from build123d import *

# Parameters (mm, degrees)
F1_DEPTH = 127
F2_R     = 33.02
F3_DEPTH = 121.92
F2_R_2   = 35.052
F4_DEPTH = 25.4
F5_R     = 2.54
F6_W     = 76.2
F6_H     = 2.54
F7_DEPTH = 5.08
F8_W     = 76.2
F8_H     = 2.54
F9_DEPTH = 5.08


with BuildPart() as f1:
    # F0 (on Top) → F1 (new body)
    with BuildSketch(Plane.XY):
        with BuildLine():
            Line((38.1, -33.553976), (18.048288, -33.553976))
            ThreePointArc((18.048288, -33.553976), (0, 38.1), (-18.048288, -33.553976))
            Line((-18.048288, -33.553976), (-38.1, -33.553976))
            Line((-38.1, -33.553976), (-38.1, -38.1))
            Line((-38.1, -38.1), (38.1, -38.1))
            Line((38.1, -38.1), (38.1, -33.553976))
        make_face()
    extrude(amount=F1_DEPTH)

    # F2 (on face) → F3 (cut)
    with BuildSketch(Plane.XY.offset(127)):
        Circle(F2_R)
    extrude(amount=-F3_DEPTH, mode=Mode.SUBTRACT)

    # F2 (on face) → F4 (join)
    with BuildSketch(Plane.XY.offset(127)):
        Circle(F2_R_2)
        Circle(F2_R, mode=Mode.SUBTRACT)
    extrude(amount=F4_DEPTH)

    # F5
    f5_edges = [f1.edges().sort_by_distance(p)[0] for p in [
        (18.048288, -33.553976, 63.5),
        (-18.048288, -33.553976, 63.5),
    ]]
    fillet(f5_edges, radius=F5_R)

    # F6 (on face) → F7 (join)
    with BuildSketch(Plane.XZ.offset(38.1)):
        with Locations((0, 1.27)):
            Rectangle(F6_W, F6_H)
    extrude(amount=F7_DEPTH)

    # F8 (on face) → F9 (join)
    with BuildSketch(Plane.XY.offset(2.54)):
        with Locations((0, -41.91)):
            Rectangle(F8_W, F8_H)
    extrude(amount=F9_DEPTH)


solid = f1.part
Geometry: final body of the model. Coordinates: model frame, mm. A direction names the side the tool comes from. Give positions to 0.01 mm unless a question says otherwise; leave off trailing zeros. Loops run counter-clockwise (first coordinate to the right, second up) from the corner with the lowest first, then second, coordinate; pieces in that order, holes last. Notation, with made-up numbers: (83, 13.5) - (125, 13.5) arc R20 ccw to (125, 41.5) - close; hole circle Ø1 at (37.5, 41.5). An arc over 180 degrees is marked (long way). One line per question, with ' | ' between items. Start each with the question number.
(1) Contact query for flat-ended pins moving along their axis: pin 1 (4 mm diameter, centred on x = -15, z = 62.5, fed in from -Y); pin 2 (3 mm diameter, centred on x = -6, y = -41.5, fed in from +Z); pin 3 (5.5 mm diameter, centred on x = 14, z = 6, fed in from +Y); pin 4 (3 mm diameter, centred on x = 3.5, y = -23.5, fed in from -Z). Output: stop coordinate, or through.
(2) Reachability of faces 1 (the flat face through (-1, -40.64, 5)), 2 (the flat face through (32, -33.554, 63)), 3 (the flat face through (0, 0, 5.08)), 4 (the flat face through (-32, -33.554, 63)) from +Z, -Z, +X, -X, +Y, -Y: full face, straight path, thin tool, end or side. Return the list, or none.
(3) Section query B-B on z = 109. Return loops of the section in (x, y).
(4) Section query A-A on x = 0. Return loops of the section in (y, z), then the cut area to 3 significant figures.
(5) Section query C-C on y = 23.5. Return loops of the section in (x, z), then the cut area to 3 significant figures.
(6) Ray query, line 1 (Y direction, x = -25, z = 108.5); line 2 (Y direction, x = 0, z = 77); line 3 (Y direction, x = -30, z = 87). Return the intervals inside material, ascending. Write a range as from..to.
(7) Section query D-D on z = 136. Return loops of the section in (x, y), then the cut area to 3 significant figures.
(8) Pull-direction query (Y, two-part tool) for faces 5 (the cylindrical face through (33.433, 10.529, 139.522)), 6 (the cylindrical face through (1.301, 38.078, 62.611)), 7 (the cylindrical face through (23.864, -31.847, 64.389)), 8 (the flat face through (-38.1, -36, 63)); classes: released by +Y, released by -Y, zero draft, split by the parting line, or undercut.
The answers:
1) pin 1: y = -38.1 | pin 2: z = 7.62 | pin 3: y = 36.4 | pin 4: z = 0
2) face 1: +Z, +X, -X | face 2: +Z, -Z, +X | face 3: +Z | face 4: +Z, -Z, -X
3) outline: (-38.1, -38.1) - (38.1, -38.1) - (38.1, -33.55) - (26.26, -33.55) arc R2.54 cw to (24.62, -29.08) arc R38.1 ccw (long way) to (-24.62, -29.08) arc R2.54 cw to (-26.26, -33.55) - (-38.1, -33.55) - close; hole circle Ø66.04 at (0, 0)
4) outline: (-43.18, 0) - (38.1, 0) - (38.1, 127) - (35.05, 127) - (35.05, 152.4) - (33.02, 152.4) - (33.02, 5.08) - (-33.02, 5.08) - (-33.02, 152.4) - (-35.05, 152.4) - (-35.05, 127) - (-38.1, 127) - (-38.1, 2.54) - (-40.64, 2.54) - (-40.64, 7.62) - (-43.18, 7.62) - close | area: 1,750 mm2
5) outline: (-29.99, 0) - (29.99, 0) - (29.99, 127) - (26.01, 127) - (26.01, 152.4) - (23.2, 152.4) - (23.2, 5.08) - (-23.2, 5.08) - (-23.2, 152.4) - (-26.01, 152.4) - (-26.01, 127) - (-29.99, 127) - close | area: 2,100 mm2
6) line 1: -38.1..-33.22, -28.75..-21.57, 21.57..28.75 | line 2: -38.1..-33.02, 33.02..38.1 | line 3: -38.1..-33.55, -23.49..-13.8, 13.8..23.49
7) outline: circle Ø70.1 at (0, 0); hole circle Ø66.04 at (0, 0) | area: 435 mm2
8) face 5: split by the parting line | face 6: undercut | face 7: undercut | face 8: zero draft
